Geometry: final body of the model. Coordinates: model frame, mm. Face numbers are marked on the shaded views. A direction names the side the tool comes from. Round coordinates to 2 decimals unless told otherwise and drop trailing zeros. Loops run counter-clockwise (first coordinate to the right, second up) from the corner with the lowest first, then second, coordinate; pieces in that order, holes last. Notation, with made-up numbers: (61.25, 67) - (70.25, 67) arc R28 cw to (70.25, 96) - close; hole circle Ø10 at (77.25, 25). An arc over 180 degrees is marked (long way). Write item = value, one per line. Start each with the question number.
Item 1: Section C-C (x = 4). Return loops of the section in (y, z), plus the area to 3 significant figures.
Item 2: Line query: line 1 (X direction, y = 6.5, z = 21.5); line 2 (X direction, y = 0, z = 1.85); line 3 (X direction, y = 5.75, z = 9.5). Output: solid intervals per line, ascending. Write a range as from..to.
Item 3: Access query for the marked faces 5 and 6. Directions: +Z, -Z, +X, -X, +Y, -Y. A direction counts if a zero-diameter tool reaches every point of the face in a straight line with its end or side. Return the directions, or none.
Item 4: Section B-B (y = 0). Count the separate pieces of the cut face and the enclosed holes in it, plus the area to 3 significant figures.
Item 5: Section D-D (z = 18). Return loops of the section in (x, y), plus the area to 3 significant figures.
Item 6: First-contact query: pin 1 (0.6 mm diameter, centred on x = -19, z = 5.5, fed in from +Y); pin 2 (10 mm diameter, centred on x = 11, y = 4.5, fed in from +Z); pin 3 (3 mm diameter, centred on y = 5, z = 27.5, fed in from +X); pin 4 (4.5 mm diameter, centred on x = 18.25, z = 21.5, fed in from +Y). Flat tips, straight axial feed; report the tip coordinate or a pass-through.
Item 7: Draft query along Z for the marked faces 1, 2, 3 and 4. Return one class per face: pulls with the +Z half, pulls with the -Z half, needs draft (parallel to the pull), parting line crosses it, or undercut.
Item 8: Section A-A (y = -3.75). Return loops of the section in (x, z).
from build123d import *
from build123d.topology import SkipClean

# Parameters (mm, degrees)
BOSS_EXTRUDE1_DEPTH      = 12
BOSS_EXTRUDE1_DEPTH_BACK = 6
SKETCH1_R                = 2.7
SKETCH3_R                = 1.7
CUT_EXTRUDE1_DEPTH       = 10
CUT_EXTRUDE2_START       = -5
CUT_EXTRUDE2_DEPTH       = 2
CUT_EXTRUDE3_DEPTH       = 10


with BuildPart() as part:
    # Sketch1 → Boss-Extrude1 (new, two sides: drawn at the far end of the back side and taken through both)
    with BuildSketch(Plane(origin=(0, 0, 0), x_dir=(1, 0, 0), z_dir=(0, 1, 0)).offset(-BOSS_EXTRUDE1_DEPTH_BACK)):
        with BuildLine():
            Line((-24.75, 0), (-24.75, -21.5))
            ThreePointArc((-24.75, -21.5), (-23.762283916, -24.944521161), (-21.099315068, -27.342208798))
            Line((-21.099315068, -27.342208798), (-6.356164384, -34.532619627))
            ThreePointArc((-6.356164384, -34.532619627), (-3.261672532, -35.628393125), (0, -36))
            Line((0, -36), (0, -27.5))
            ThreePointArc((0, -27.5), (-6, -21.5), (0, -15.5))
            Line((0, -15.5), (0, 0))
            Line((0, 0), (-24.75, 0))
        make_face()
        with Locations(Location((-18.25, -21.5, 0), (0, 0, 270))):
            Circle(SKETCH1_R, mode=Mode.SUBTRACT)
    extrude(amount=BOSS_EXTRUDE1_DEPTH + BOSS_EXTRUDE1_DEPTH_BACK)

    # Sketch3 → Cut-Extrude1 (cut)
    with BuildSketch(Plane(origin=(0, 0, 0), x_dir=(-1, 0, 0), z_dir=(0, 0, -1))):
        with Locations((18.75, 6)):
            Circle(SKETCH3_R)
        with BuildLine():
            Line((0, 1.7), (0, -1.7))
            ThreePointArc((0, -1.7), (1.7, 0), (0, 1.7))
        make_face()
    extrude(amount=-CUT_EXTRUDE1_DEPTH, mode=Mode.SUBTRACT)

    # Sketch4 → Cut-Extrude2 (cut)
    with BuildSketch(Plane(origin=(0, 0, 0), x_dir=(-1, 0, 0), z_dir=(0, 0, -1)).offset(CUT_EXTRUDE2_START)):
        Polygon((15.75, 9), (15.75, 12), (21.75, 12), (21.75, 9), (21.75, 3), (15.75, 3), align=None)
        Polygon((0, 3), (3, 3), (3, 0), (3, -6), (0, -6), align=None)
    extrude(amount=-CUT_EXTRUDE2_DEPTH, mode=Mode.SUBTRACT)

    # Sketch6 → Cut-Extrude3 (cut)
    with BuildSketch(Plane.XZ.offset(6)):
        Polygon((-14, 23.953738644), (-18.25, 26.407477288), (-22.5, 23.953738644), (-22.5, 19.046261356), (-18.25, 16.592522712), (-14, 19.046261356), align=None)
    extrude(amount=-CUT_EXTRUDE3_DEPTH, mode=Mode.SUBTRACT)

    # Mirror1: part across plane


with BuildPart() as part_1:
    with SkipClean():  # the faces are left unmerged after this step: merging them gives an invalid solid
        add(part.part)
        add(part.part.mirror(Plane(origin=(0, -6, 0), x_dir=(0, 0, 1), z_dir=(1, 0, 0))))


solid = part_1.part
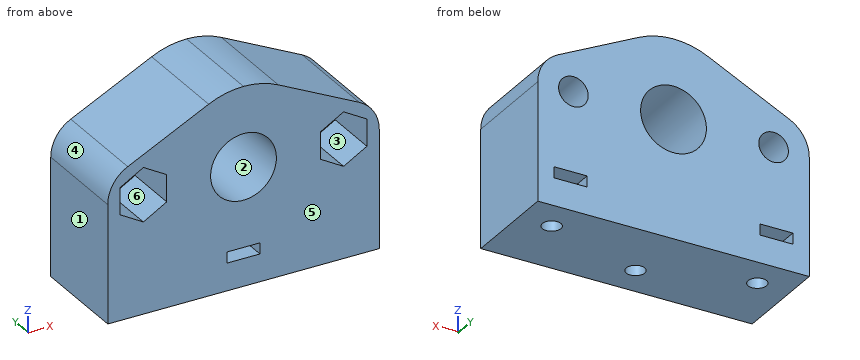
Taken from the geometry:
q1.outline = (-6, 0) - (12, 0) - (12, 17.03) - (-6, 17.03) - close; (-6, 25.97) - (12, 25.97) - (12, 35.44) - (-6, 35.44) - close
q1.area = 477 mm^2
q2.line_1 = -24.75..-20.95, -15.55..-6, 6..15.55, 20.95..24.75
q2.line_2 = -24.75..-1.7, 1.7..24.75
q2.line_3 = -24.75..-20.43, -17.07..17.07, 20.43..24.75
q3.face_5 = +Z, -Z, +X, -X, -Y
q3.face_6 = -Y
q4.separate_pieces = 1
q4.enclosed_holes = 3
q4.area = 1,270 mm^2
q5.outline = (-24.75, -6) - (-20.69, -6) - (-20.69, 4) - (-15.81, 4) - (-15.81, -6) - (-4.87, -6) - (-4.87, 12) - (-24.75, 12) - close; (4.87, -6) - (15.81, -6) - (15.81, 4) - (20.69, 4) - (20.69, -6) - (24.75, -6) - (24.75, 12) - (4.87, 12) - close
q5.area = 618 mm^2
q6.pin_1 = 3
q6.pin_2 = 34.7
q6.pin_3 = 22.94
q6.pin_4 = through
q7.face_1 = needs draft
q7.face_2 = undercut
q7.face_3 = undercut
q7.face_4 = pulls with the +Z half
q8.outline = (-24.75, 0) - (24.75, 0) - (24.75, 21.5) arc R6.5 ccw to (21.1, 27.34) - (6.36, 34.53) arc R14.5 ccw to (-6.36, 34.53) - (-21.1, 27.34) arc R6.5 ccw to (-24.75, 21.5) - close; hole (-22.5, 19.05) - (-18.25, 16.59) - (-14, 19.05) - (-14, 23.95) - (-18.25, 26.41) - (-22.5, 23.95) - close; hole circle Ø12 at (0, 21.5); hole (-3, 5) - (3, 5) - (3, 7) - (-3, 7) - close; hole (14, 19.05) - (18.25, 16.59) - (22.5, 19.05) - (22.5, 23.95) - (18.25, 26.41) - (14, 23.95) - close
